Verification items for the finished model (mm, model axes). Coordinates: 2 decimals unless noted, no trailing zeros. Order: outer loops, then holes, each group sorted by start corner. A loop starts at its lowest first (then second) coordinate and runs counter-clockwise, first axis right, second up. Notation, with made-up numbers: M 36.5,62 L 52.5,62 A26 ccw 52.5,84 Z; hole C 24,-20.5 d9. An arc over 180 degrees is marked long. Return JSON: item names as keys, results as strings.
Autodesk Inventor part; units mm, degrees
ref_plane "YZ Plane" through (0, 0, 0) normal (1, 0, 0) x (0, 1, 0)
ref_plane "XZ Plane" through (0, 0, 0) normal (0, 1, 0) x (-1, 0, 0)
ref_plane "XY Plane" through (0, 0, 0) normal (0, 0, 1) x (1, 0, 0)
sketch "Sketch1" plane through (0, 0, 0) normal (0, 0, 1) x (1, 0, 0)
  line L0 (-25.5, -25.5) -> (25.5, -25.5)
  line L1 (25.5, -25.5) -> (25.5, 25.5)
  line L2 (25.5, 25.5) -> (-25.5, 25.5)
  line L3 (-25.5, 25.5) -> (-25.5, -25.5)
  line L4 (-25.5, -25.5) -> (25.5, 25.5) construction
  line L5 (25.5, -25.5) -> (-25.5, 25.5) construction
  point P0 (0, 0)
  dimension "d0" = 51
  dimension "d1" = 51
extrude "Extrusion1" add sketch "Sketch1" against normal blind 2.921
sketch "Sketch2" plane through (0, 0, 0) normal (0, 0, 1) x (1, 0, 0)
  line L0 (-13.0551, 25.5) -> (-9.5, 25.5)
  line L1 (-9.5, 25.5) -> (-9.5, 22.5)
  line L2 (-9.5, 22.5) -> (9.5, 22.5)
  line L3 (9.5, 22.5) -> (9.5, 25.5)
  line L4 (-9.5, 25.5) -> (9.5, 25.5)
  line L5 (-9.5, -25.5) -> (9.5, -25.5)
  line L6 (9.5, -25.5) -> (9.5, -22.5)
  line L7 (9.5, -22.5) -> (-9.5, -22.5)
  line L8 (-9.5, -22.5) -> (-9.5, -25.5)
  line L9 (-25.5, 9.5) -> (-22.5, 9.5)
  line L10 (-22.5, 9.5) -> (-22.5, -9.5)
  line L11 (-22.5, -9.5) -> (-25.5, -9.5)
  line L12 (-25.5, -9.5) -> (-25.5, 9.5)
  line L13 (25.5, 9.5) -> (22.5, 9.5)
  line L14 (22.5, 9.5) -> (22.5, -9.5)
  line L15 (22.5, -9.5) -> (25.5, -9.5)
  line L16 (25.5, -9.5) -> (25.5, 9.5)
  line L17 (25.5, -25.5) -> (25.5, 25.5)
  line L18 (-25.5, 25.5) -> (-25.5, -25.5)
  line L19 (-25.5, -25.5) -> (25.5, -25.5)
  line L20 (25.5, 25.5) -> (-25.5, 25.5)
  line L21 (-25.5, 25.5) -> (-25.5, -25.5)
  dimension "d4" = 3
  dimension "d5" = 19
  dimension "d17" = 19
  dimension "d18" = 3
  dimension "d19" = 3
  dimension "d20" = 19
  dimension "d34" = 3
  dimension "d35" = 19
  dimension "d47" = 16
  dimension "d48" = 16
  dimension "d49" = 16
  dimension "d50" = 16
  dimension "d51" = 16
  dimension "d52" = 45
extrude "Extrusion3" cut sketch "Sketch2" against normal blind 25.4 contours L4 L3 L2 L1 | L9 L10 L11 L12 | L16 L15 L14 L13 | L8 L7 L6 L5
hole "Hole1" at (-0.1, 0, 0) direction (0, 0, -1) diameter 25.4 end through all
equation "\"d1\" = d0"
equation "\"d17\" = d5"
equation "\"d18\" = d4"
equation "\"d19\" = d4"
equation "\"d20\" = d5"
equation "\"d34\" = d4"
equation "\"d35\" = d5"
equation "\"d47\" = -0.5 * d5 + 0.5 * d0"
equation "\"d49\" = d47"
equation "\"d50\" = d47"
equation "\"d51\" = d47"
equation "\"d53\" = 0.5 * d0"
properties part number "Side A"
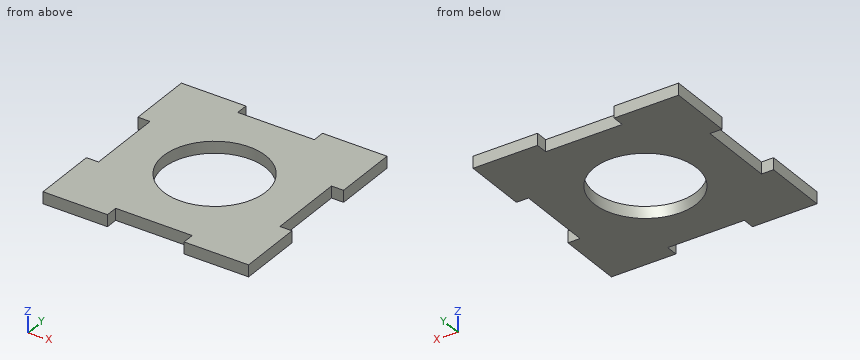
Q1. Material ranges on line 1 along X through (y, z) = (0.5, -0.35); line 2 along Y through (x, z) = (-0.1, -0.9); line 3 along X through (y, z) = (10, -1.3), recorded low to high.
Values:
{"line 1": "-22.5 to -12.79, 12.59 to 22.5", "line 2": "-22.5 to -12.7, 12.7 to 22.5", "line 3": "-25.5 to -7.93, 7.73 to 25.5"}
Q2. Cross-section at B-B, the plane x = -0.1. Record the boundary of the cut face in (y, z), and give its area (3 significant figures).
Values:
{"outline": "M -22.5,-2.92 L -12.7,-2.92 L -12.7,0 L -22.5,0 Z; M 12.7,-2.92 L 22.5,-2.92 L 22.5,0 L 12.7,0 Z", "area": "57.3 mm^2"}
Q3. Cross-section at A-A, the plane y = 0. Record the boundary of the cut face in (x, z), and give its area (3 significant figures).
Values:
{"outline": "M -22.5,-2.92 L -12.8,-2.92 L -12.8,0 L -22.5,0 Z; M 12.6,-2.92 L 22.5,-2.92 L 22.5,0 L 12.6,0 Z", "area": "57.3 mm^2"}
Q4. Cross-section at C-C, the plane z = -2.05. Record the boundary of the cut face in (x, y).
Values:
{"outline": "M -25.5,-25.5 L -9.5,-25.5 L -9.5,-22.5 L 9.5,-22.5 L 9.5,-25.5 L 25.5,-25.5 L 25.5,-9.5 L 22.5,-9.5 L 22.5,9.5 L 25.5,9.5 L 25.5,25.5 L 9.5,25.5 L 9.5,22.5 L -9.5,22.5 L -9.5,25.5 L -25.5,25.5 L -25.5,9.5 L -22.5,9.5 L -22.5,-9.5 L -25.5,-9.5 Z; hole C -0.1,0 d25.4"}
Q5. Go/stop test with a flat-tipped pin: pin 1 (1.5 mm diameter, centred on y = -1.5, z = -1.5, fed in from +X). Record where the tip stops, or that it passes through.
Values:
{"pin 1": "x = 22.5"}
